Could you check a few things on this model? Use its own coordinates, in mm. Face numbers are marked on the shaded views. A direction names the side the tool comes from. Round coordinates to 2 decimals unless told otherwise and drop trailing zeros. Loops run counter-clockwise (first coordinate to the right, second up) from the corner with the lowest first, then second, coordinate; pieces in that order, holes last. Notation, with made-up numbers: (1, -3.5) -> (19, -3.5) arc R27 ccw to (19, 15.5) -> close; hole circle Ø6 at (83.5, 47.25). An arc over 180 degrees is marked (long way). Write each question's results on one line, items separated by ' | '.
from build123d import *

# Parameters (mm, degrees)
SKETCH_1_R          = 4
SKETCH_1_R_2        = 4.1
EXTRUDE_1_DEPTH     = 15.875
CHAMFER_1_SIZE      = 2
SKETCH_2_R          = 4.5
CUT_EXTRUDE_1_DEPTH = 20
SKETCH_3_R          = 4.5
CUT_EXTRUDE_2_DEPTH = 20
CHAMFER_2_SIZE      = 20
CHAMFER_3_SIZE      = 10
FILLET_1_R          = 10


with BuildPart() as part:
    # 草图1 → 凸台-拉伸1 (new body)
    with BuildSketch(Plane.XY):
        Polygon((0, 10), (-130, 10), (-130, -20), (-110, -20), (-110, -10), (0, -10), (65, -10), (65, -30), (85, -30), (85, 10), align=None)
        Circle(SKETCH_1_R, mode=Mode.SUBTRACT)
        with Locations((-30, 0)):
            Circle(SKETCH_1_R_2, mode=Mode.SUBTRACT)
        with Locations((75, 0)):
            Circle(SKETCH_1_R_2, mode=Mode.SUBTRACT)
        with Locations((75, -20)):
            Circle(SKETCH_1_R_2, mode=Mode.SUBTRACT)
        with Locations((-120, -10)):
            Circle(SKETCH_1_R_2, mode=Mode.SUBTRACT)
    extrude(amount=EXTRUDE_1_DEPTH)

    # 倒角1
    chamfer_1_edges = [part.edges().sort_by_distance(p)[0] for p in [
        (-130, 10, 7.9375),
        (85, 10, 7.9375),
        (85, -30, 7.9375),
        (-130, -20, 7.9375),
    ]]
    chamfer(chamfer_1_edges, length=CHAMFER_1_SIZE)

    # 草图2 → 切除-拉伸1 (cut)
    with BuildSketch(Plane(origin=(0, 0, 0), x_dir=(-1, 0, 0), z_dir=(0, 0, -1))):
        with Locations((-30, 0)):
            Circle(SKETCH_2_R)
    extrude(amount=-CUT_EXTRUDE_1_DEPTH, mode=Mode.SUBTRACT)

    # 草图3 → 切除-拉伸2 (cut)
    with BuildSketch(Plane(origin=(0, 0, 0), x_dir=(-1, 0, 0), z_dir=(0, 0, -1))):
        with Locations((80, 0)):
            Circle(SKETCH_3_R)
    extrude(amount=-CUT_EXTRUDE_2_DEPTH, mode=Mode.SUBTRACT)

    # 倒角2
    chamfer_2_edges = [part.edges().sort_by_distance(p)[0] for p in [
        (65, -10, 7.9375),
    ]]
    chamfer(chamfer_2_edges, length=CHAMFER_2_SIZE - 0.0001)  # a hair under: the kernel refuses the full size

    # 倒角3
    chamfer_3_edges = [part.edges().sort_by_distance(p)[0] for p in [
        (-110, -10, 7.9375),
    ]]
    chamfer(chamfer_3_edges, length=CHAMFER_3_SIZE - 0.0001)  # a hair under: the kernel refuses the full size

    # 圆角1
    fillet_1_edges = [part.edges().sort_by_distance(p)[0] for p in [
        (45.0001, -10, 7.9375),
        (-100.0001, -10, 7.9375),
    ]]
    fillet(fillet_1_edges, radius=FILLET_1_R)


solid = part.part
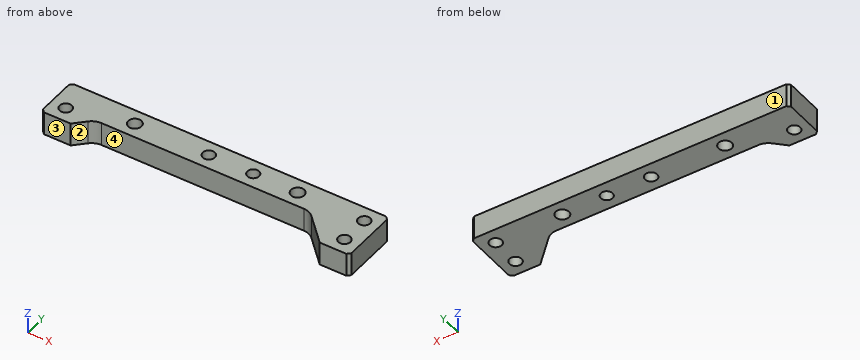
1) For the marked faces 1 and 2, which set-ups out of +Z, -Z, +X, -X, +Y, -Y let a thin tool reach every point of the face, with its end or its side?
Model answer:
face 1: +Z, -Z, +X, -X, +Y | face 2: +Z, -Z, -Y
2) I want a section at B-B, the plane x = 30. Write out the boundary of the cut face in (y, z) (3 decimals).
Model answer:
outline: (-10, 0) -> (-4.5, 0) -> (-4.5, 15.875) -> (-10, 15.875) -> close; (4.5, 0) -> (10, 0) -> (10, 15.875) -> (4.5, 15.875) -> close
3) I want a section at A-A, the plane z = 5.5. Give the number of separate pieces and of enclosed holes in the cut face, plus the area to 3 significant figures.
Model answer:
separate pieces: 1 | enclosed holes: 7 | area: 4,760 mm2
4) If we mould it in two halves opening along X, with no side actions, what happens to the marked faces 3 and 4? For each: released by +X, released by -X, zero draft, split by the parting line, or undercut.
Model answer:
face 3: zero draft | face 4: undercut
5) I'm going to push flat-ended pins straight in: pin 1 (13 mm diameter, centred on x = -30, y = 0, fed in from -Z); pin 2 (8 mm diameter, centred on y = -24.5, z = 7, fed in from -X); pin 3 (8 mm diameter, centred on x = 51.5, z = 3.5, fed in from -Y). Where does each tip first touch, or does it pass through?
Model answer:
pin 1: stops at z = 0 | pin 2: stops at x = 55.5 | pin 3: stops at y = -20.5
6) I want a section at C-C, the plane x = -24. Write out the boundary of the cut face in (y, z) (3 decimals).
Model answer:
outline: (-10, 0) -> (10, 0) -> (10, 15.875) -> (-10, 15.875) -> close
7) I need wall thicknesses on line 1 (Y direction, x = -120, z = 5.75); line 2 (X direction, y = -13, z = 4.25); line 3 (X direction, y = -1, z = 5.5). Which ranges of each line are inside material? Lowest first, please.
Model answer:
line 1: y = -20 to -14.1, -5.9 to 10 | line 2: x = -130 to -122.79, -117.21 to -103, 48 to 85 | line 3: x = -130 to -84.39, -75.61 to -33.98, -26.02 to -3.87, 3.87 to 25.61, 34.39 to 71.02, 78.98 to 85
